Input: part model. Units: mm. Frame: model coordinates. Give positions to 0.01 mm unless a question says otherwise; leave off trailing zeros. One line per question, with ' | ' between items.
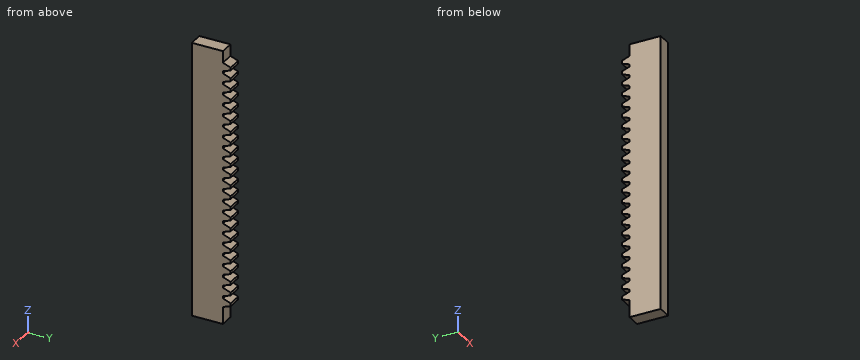
from build123d import *

# Parameters (mm, degrees)
SKETCH1_W           = 18
SKETCH1_H           = 160
BOSS_EXTRUDE1_DEPTH = 8
BOSS_EXTRUDE2_DEPTH = 8
LPATTERN1_COUNT     = 23
LPATTERN1_PITCH     = 6.283


with BuildPart() as part:
    # Sketch1 → Boss-Extrude1 (new body)
    with BuildSketch(Plane.YZ):
        Rectangle(SKETCH1_W, SKETCH1_H)
    extrude(amount=BOSS_EXTRUDE1_DEPTH)

    # Sketch2 → Boss-Extrude2 (add)
    with BuildSketch(Plane.YZ):
        Polygon((9, -70), (9, -65.04), (13.5, -66.675), (13.5, -67.52), (13.5, -68.365), align=None)
    boss_extrude2 = extrude(amount=BOSS_EXTRUDE2_DEPTH)

    # LPattern1: Boss-Extrude2 ×23
    with Locations(*[(0, 0, i * LPATTERN1_PITCH) for i in range(1, LPATTERN1_COUNT)]):
        add(boss_extrude2)


solid = part.part
1. Pin query (flat end, axial travel): P1, Ø0.7, axis at x = 3.5, z = -39, coming from the +Y side; P2, Ø1.5, axis at x = 2, y = 10.5, coming from the -Z side. Return the tip coordinate at first contact, or that it passes through.
Determined:
P1: stops at y = 9 | P2: stops at z = -69.73
2. Ray query, line 1 along Y through (x, z) = (1.5, -14.5). Return the intervals inside material, ascending. Write a range as from..to.
Determined:
line 1: y = -9..9
3. Section query A-A (y = 11). Count the separate pieces of the cut face and the enclosed holes in it, then the cut area to 3 significant figures.
Determined:
separate pieces: 23 | enclosed holes: 0 | area: 645 mm2
